For this review, take the finished solid that the model builds, in its own axes (mm). Give positions to 0.01 mm unless a question says otherwise; leave off trailing zeros. Loops run counter-clockwise (first coordinate to the right, second up) from the corner with the lowest first, then second, coordinate; pieces in that order, holes last. Notation, with made-up numbers: (72.25, -36.5) -> (115.25, -36.5) arc R22 ccw to (115.25, -19.5) -> close; hole circle Ø2 at (16, 41.25). An arc over 180 degrees is marked (long way). Write each question's results on one line, items separated by ' | '. Start each with the question number.
```python
from build123d import *

# Parameters (mm, degrees)
SKETCH1_W           = 25.4
SKETCH1_H           = 25.4
BOSS_EXTRUDE1_DEPTH = 133.4008
SKETCH2_R           = 6.524301876
CUT_EXTRUDE2_DEPTH  = 26.4
CUT_EXTRUDE3_DEPTH  = 26.4


with BuildPart() as part:
    # Sketch1 → Boss-Extrude1 (new body)
    with BuildSketch(Plane.XY):
        Rectangle(SKETCH1_W, SKETCH1_H)
    extrude(amount=-BOSS_EXTRUDE1_DEPTH)

    # Sketch2 → Cut-Extrude2 (cut, through all)
    with BuildSketch(Plane(origin=(0, 12.7, 0), x_dir=(1, 0, 0), z_dir=(0, 1, 0))):
        with Locations((0, 76.2)):
            Circle(SKETCH2_R)
    extrude(amount=-CUT_EXTRUDE2_DEPTH, mode=Mode.SUBTRACT)

    # Sketch3 → Cut-Extrude3 (cut, through all)
    with BuildSketch(Plane(origin=(0, 12.7, 0), x_dir=(1, 0, 0), z_dir=(0, 1, 0))):
        Polygon((12.7, 133.4008), (6.96541308, 133.4008), (12.7, 23.978363128), align=None)
    extrude(amount=-CUT_EXTRUDE3_DEPTH, mode=Mode.SUBTRACT)


solid = part.part
```
1. Draft analysis for pull direction X (two halves, no side actions). For faces 1 (the flat face through (9.793, 0.178, -79.456)), 2 (the flat face through (0, -12.7, -66)), 3 (the cylindrical face through (-1.41, 0.18, -69.83)), state which applies: released by +X, released by -X, zero draft, split by the parting line, or undercut.
2. We need section B-B (y = 1). Write out the cut boundary in (x, z), plus the area to 3 significant figures.
3. For pin 1 Ø1 at (y, z) = (-1, -99.5) entering from +X, flat-tipped, find the tip position at first contact; note if it passes through.
4. Wall thickness on L1, parallel to Z at x = 0, y = -7; L2, parallel to Z at x = -3.25, y = 5.5; L3, parallel to X at y = 3.75, z = -76.2: over which ranges is each line inside the solid? List them lowest first.
5. We need section D-D (z = -108). Write out the cut boundary in (x, y), plus the area to 3 significant figures.
6. We need section C-C (x = 0). Write out the cut boundary in (y, z), plus the area to 3 significant figures.
7. We need section A-A (z = -76.2). Write out the cut boundary in (x, y), plus the area to 3 significant figures.
Response:
1) face 1: released by +X | face 2: zero draft | face 3: undercut
2) outline: (-12.7, -133.4) -> (6.97, -133.4) -> (12.7, -23.98) -> (12.7, 0) -> (-12.7, 0) -> close; hole circle Ø13.05 at (0, -76.2) | area: 2,940 mm2
3) pin 1: stops at x = 8.77
4) L1: z = -133.4 to -82.72, -69.68 to 0 | L2: z = -133.4 to -81.86, -70.54 to 0 | L3: x = -12.7 to -6.52, 6.52 to 9.96
5) outline: (-12.7, -12.7) -> (8.3, -12.7) -> (8.3, 12.7) -> (-12.7, 12.7) -> close | area: 533 mm2
6) outline: (-12.7, -133.4) -> (12.7, -133.4) -> (12.7, -82.72) -> (-12.7, -82.72) -> close; (-12.7, -69.68) -> (12.7, -69.68) -> (12.7, 0) -> (-12.7, 0) -> close | area: 3,060 mm2
7) outline: (-12.7, -12.7) -> (-6.52, -12.7) -> (-6.52, 12.7) -> (-12.7, 12.7) -> close; (6.52, -12.7) -> (9.96, -12.7) -> (9.96, 12.7) -> (6.52, 12.7) -> close | area: 244 mm2
